```python
from build123d import *

# Parameters (mm, degrees)
F1_R    = 13.1633
F1_R_2  = 11.1633
F3_SIZE = 0.635
F4_R    = 0.508


with BuildPart() as f2:
    # F2: sweep along a path in F0
    with BuildLine(Plane.XY) as f2_path:
        Line((-21.9970452561, -12.7), (-6.35, -3.6661742094))
        ThreePointArc((-6.35, -3.6661742094), (0, -1.9646968374), (6.35, -3.6661742094))
        Line((6.35, -3.6661742094), (21.9970452561, -12.7))
    # F1 (on Right) → F2 (sweep)
    with BuildSketch(Plane.YZ):
        Circle(F1_R)
        Circle(F1_R_2, mode=Mode.SUBTRACT)
    sweep(path=f2_path.line)

    # F3
    f3_edges = [f2.edges().sort_by_distance(p)[0] for p in [
        (17.397744, -20.666224, 0),
        (-17.397744, -20.666224, 0),
    ]]
    chamfer(f3_edges, length=F3_SIZE)

    # F4
    f4_edges = [f2.edges().sort_by_distance(p)[0] for p in [
        (-17.080244, -21.21615, 0),
        (-16.847818, -20.348724, 0),
        (16.847818, -20.348724, 0),
        (17.080244, -21.21615, 0),
    ]]
    fillet(f4_edges, radius=F4_R)


solid = f2.part
```
The listing builds one solid part. Answer for the finished solid, in the listing's coordinates (mm). Round coordinates to 2 decimals unless told otherwise and drop trailing zeros.
1) Given P1, Ø3, axis at x = 8.5, y = -16, coming from the -Z side; P2, Ø1, axis at x = 18.5, z = 8.5, coming from the +Y side; P3, Ø2, axis at x = -22, z = 3.5, coming from the +Y side; P4, Ø1, axis at y = -2, z = -1.5, coming from the -X side, each flat-ended and moving along its own axis, determine where each tip first touches the part or whether it passes through.
Outcome:
P1: stops at z = -8.48
P2: stops at y = 3.74
P3: stops at y = 4.87
P4: passes through
2) For a pull along Y with two mould halves and no side action, classify faces 1 (the face through (-24.9, -7.67, -11.64)), 2 (the face through (-21.324, 4.455, 3.954)), 3 (the face through (20.05, 2.6, -4.28)) as released by +Y, released by -Y, zero draft, split by the parting line, or undercut.
Outcome:
face 1: released by -Y
face 2: split by the parting line
face 3: undercut
3) Consider line 1 (Z direction, x = 17, y = -7); line 2 (Y direction, x = -1.5, z = -10); line 3 (Y direction, x = -1.5, z = 1.5). Determine where each line is inside the solid, lowest interval first.
Outcome:
line 1: z = -13.15 to -11.15, 11.15 to 13.15
line 2: y = -8.75 to -5.08, 4.9 to 8.51
line 3: y = -13.7 to -11.39, 11.02 to 13.04
